```python
from build123d import *

# Parameters (mm, degrees)
SKETCH1_R           = 6
SKETCH1_R_2         = 1.1303
SKETCH1_R_3         = 3.175
SKETCH1_R_4         = 1.524
BOSS_EXTRUDE1_DEPTH = 6.35
FILLET1_R           = 5


with BuildPart() as part:
    # Sketch1 → Boss-Extrude1 (new body)
    with BuildSketch(Plane.XY):
        with BuildLine():
            Line((-50.8, 10.7), (-50.8, -10.7))
            ThreePointArc((-50.8, -10.7), (-50.214213562, -12.114213562), (-48.8, -12.7))
            Line((-48.8, -12.7), (0, -12.7))
            Line((0, -12.7), (17.940725429, -23.578549747))
            ThreePointArc((17.940725429, -23.578549747), (17.571857186, -25.980430432), (19.009414234, -27.939645668))
            Line((19.009414234, -27.939645668), (40.728550204, -41.109274848))
            ThreePointArc((40.728550204, -41.109274848), (43.130430599, -41.478142773), (45.089645569, -40.040585929))
            Line((45.089645569, -40.040585929), (58.259274749, -18.321449959))
            ThreePointArc((58.259274749, -18.321449959), (58.628143126, -15.91957084), (57.1905883, -13.960355869))
            Line((57.1905883, -13.960355869), (35.47145233, -0.790726689))
            ThreePointArc((35.47145233, -0.790726689), (33.069571007, -0.421856833), (31.110354609, -1.859413778))
            Line((31.110354609, -1.859413778), (7.099208724, 12.7))
            Line((7.099208724, 12.7), (-48.8, 12.7))
            ThreePointArc((-48.8, 12.7), (-50.214213562, 12.114213562), (-50.8, 10.7))
        make_face()
        with Locations((38.1, -20.95)):
            Circle(SKETCH1_R, mode=Mode.SUBTRACT)
        with Locations((43.038610942, -12.805324011)):
            Circle(SKETCH1_R_2, mode=Mode.SUBTRACT)
        with Locations((33.161389058, -29.094675989)):
            Circle(SKETCH1_R_2, mode=Mode.SUBTRACT)
        with Locations((-6.35, 0)):
            Circle(SKETCH1_R_3, mode=Mode.SUBTRACT)
        with Locations((-25.4, 0)):
            Circle(SKETCH1_R_3, mode=Mode.SUBTRACT)
        with Locations((-44.45, 0)):
            Circle(SKETCH1_R_3, mode=Mode.SUBTRACT)
        with Locations((33.825246605, -3.505617425)):
            Circle(SKETCH1_R_4, mode=Mode.SUBTRACT)
        with Locations((20.655617425, -25.224753395)):
            Circle(SKETCH1_R_4, mode=Mode.SUBTRACT)
        with Locations((42.374753395, -38.394382575)):
            Circle(SKETCH1_R_4, mode=Mode.SUBTRACT)
        with Locations((55.544382575, -16.675246605)):
            Circle(SKETCH1_R_4, mode=Mode.SUBTRACT)
    extrude(amount=BOSS_EXTRUDE1_DEPTH)

    # Fillet1
    fillet1_edges = [part.edges().sort_by_distance(p)[0] for p in [
        (17.940725429, -23.578549747, 3.175),
        (0, -12.7, 3.175),
        (7.099208724, 12.7, 3.175),
        (31.110354609, -1.859413778, 3.175),
    ]]
    fillet(fillet1_edges, radius=FILLET1_R)


solid = part.part
```
Geometry check sheet. Reference: the model listing, model coordinates, mm. A direction names the side the tool comes from. Give positions to 0.01 mm unless a question says otherwise; leave off trailing zeros. Loops run counter-clockwise (first coordinate to the right, second up) from the corner with the lowest first, then second, coordinate; pieces in that order, holes last. Notation, with made-up numbers: M 32.25,-15.75 L 74.25,-15.75 A29 ccw 74.25,8.25 Z; hole C 40,24 d10. An arc over 180 degrees is marked long. Write item = value, one per line. Start each with the question number.
1. Section check C-C, the plane x = 38.1. Enter the section's corners in (y, z), plus the area to 3 significant figures.
2. Section check A-A, the plane x = -6.35. Enter the section's corners in (y, z) (3 decimals), plus the area to 3 significant figures.
3. Draft check along Y on faces 1 (the face through (29.717, -34.432, 3.131)), 2 (the face through (46.483, -7.468, 3.131)), 3 (the face through (42.04, -39.88, 3.13)), 4 (the face through (3, -8, 0)). Enter one of: +Y half, -Y half, draft (parallel to the pull), parting line (faces both ways), or undercut.
4. Go/stop test with flat-tipped pins: P1, Ø2.5, axis at x = 33.16, y = -29.09, coming from the +Z side; P2, Ø1, axis at x = -15, z = 2, coming from the -Y side; P3, Ø3, axis at y = -19.5, z = 1.5, coming from the -X side. Record where each tip stops, or that it passes through.
5. Thickness scan on probe 1 along Y at (x, z) = (-25.4, 3.5) (3 decimals); probe 2 along X at (y, z) = (-24, 5); probe 3 along X at (y, z) = (-16, 2.5). Record the ranges inside material, lowest first.
6. Section check B-B, the plane z = 4.75. Give the number of separate pieces and of enclosed holes in the cut face, plus the area to 3 significant figures.
7. Tool access check on faces 5 (the face through (56.95, -17.26, 3.13)), 6 (the face through (-25, -12.7, 3)). Record the directions out of +Z, -Z, +X, -X, +Y, -Y that give a thin tool (end or side, any length) a straight path to the whole face; none if there is none.
Values follow:
q1.outline = M -39.52,0 L -26.95,0 L -26.95,6.35 L -39.52,6.35 Z; M -14.95,0 L -2.38,0 L -2.38,6.35 L -14.95,6.35 Z
q1.area = 160 mm^2
q2.outline = M -12.7,0 L -3.175,0 L -3.175,6.35 L -12.7,6.35 Z; M 3.175,0 L 12.7,0 L 12.7,6.35 L 3.175,6.35 Z
q2.area = 121 mm^2
q3.face_1 = -Y half
q3.face_2 = +Y half
q3.face_3 = undercut
q3.face_4 = draft
q4.P1 = 6.35
q4.P2 = -12.7
q4.P3 = 8.74
q5.probe_1 = -12.7 to -3.175, 3.175 to 12.7
q5.probe_2 = 17.05 to 19.75, 21.56 to 32.93, 43.27 to 54.82
q5.probe_3 = 5.44 to 34.71, 41.49 to 54.18, 56.91 to 58.65
q6.separate_pieces = 1
q6.enclosed_holes = 10
q6.area = 2,760 mm^2
q7.face_5 = +Z, -Z
q7.face_6 = +Z, -Z, -X, -Y
